Build history of the part. All positions in model axes, mm. A direction names the side the tool comes from. Give positions to 0.01 mm unless a question says otherwise; leave off trailing zeros. Write each loop counter-clockwise with the first axis right and the second up, starting at its lowest first coordinate (ties: lowest second). Pieces come first, ordered by that corner, then holes.
Autodesk Inventor part; units mm, degrees
ref_plane "YZ Plane" through (0, 0, 0) normal (1, 0, 0) x (0, 1, 0)
ref_plane "XZ Plane" through (0, 0, 0) normal (0, 1, 0) x (-1, 0, 0)
ref_plane "XY Plane" through (0, 0, 0) normal (0, 0, 1) x (1, 0, 0)
sketch "Sketch1" plane through (0, 0, 0) normal (1, 0, 0) x (0, 1, 0)
  line L0 (0, 0) -> (5, 0)
  line L1 (5, 0) -> (5, 20)
  line L2 (5, 20) -> (0, 20)
  line L3 (0, 20) -> (0, 0)
  line L4 (-25, 100) -> (-30, 100)
  line L5 (-30, 100) -> (-30, 120)
  line L6 (-30, 120) -> (-25, 120)
  line L7 (-25, 120) -> (-25, 100)
  line L8 (5, 20) -> (-25, 100)
  line L9 (0, 20) -> (-30, 100)
  dimension "d0" = 5
  dimension "d1" = 20
  dimension "d2" = 5
  dimension "d3" = 20
  dimension "d4" = 35
  dimension "d5" = 120
extrude "Extrusion1" add sketch "Sketch1" along normal blind 40
sketch "Sketch2" plane through (0, 0, 0) normal (0, -1, 0) x (1, 0, 0)
  circle A0 centre (30, 10) radius 2.5
  circle A1 centre (10, 10) radius 2.5
  circle A2 centre (30, 110) radius 2.5
  circle A3 centre (10, 110) radius 2.5
  line L0 (40, 120) -> (40, 100)
  line L1 (0, 120) -> (40, 120)
  line L2 (0, 120) -> (0, 100)
  line L3 (0, 20) -> (0, 0)
  line L4 (40, 20) -> (40, 0)
  line L5 (0, 0) -> (40, 0)
  dimension "d8" = 5
  dimension "d9" = 5
  dimension "d10" = 5
  dimension "d11" = 5
  dimension "d12" = 10
  dimension "d13" = 10
  dimension "d14" = 10
  dimension "d15" = 10
  dimension "d16" = 10
  dimension "d17" = 10
  dimension "d18" = 10
  dimension "d19" = 10
extrude "Extrusion2" cut sketch "Sketch2" against normal mid plane 90
properties part number "BracketControlPannel"
1. Saw through at B-B on z = 10. Give the cut face in (x, y).
2. Drop a flat-ended pin along its axis: pin 1 (22 mm diameter, centred on x = 28.5, z = 6, fed in from -Y). Give the stop position or say it passes through.
3. Drill centre lines: line 1 along Y through (x, z) = (4, 17); line 2 along Y through (x, z) = (34, 103.5). Where is each one in solid material? Low to high.
4. Mould opens along Z. For faces 4 (the face through (20, 2, 0)), 5 (the face through (29.46, 2.46, 7.56)), 6 (the face through (9.46, 2.46, 7.56)), 7 (the face through (0, -13, 60)) say: pulls with the +Z half, pulls with the -Z half, needs draft (parallel to the pull), parting line crosses it, or undercut.
5. Saw through at C-C on x = 24. Give the cut face in (y, z).
6. Saw through at A-A on x = 30. Give the cut face in (y, z), plus the area to 3 significant figures.
7. 3-axis set-ups, long thin cutter, end or side, ignore diameter. For faces 1 (the face through (40, -13, 60)), 2 (the face through (20, 0, 10)), 3 (the face through (20, -25, 110)): which of +Z, -Z, +X, -X, +Y, -Y reach the whole face in a straight line?
8. Saw through at D-D on z = 96.5. Give the cut face in (x, y).
Outcome:
1. outline: (0, 0) - (7.5, 0) - (7.5, 5) - (0, 5) - close; (12.5, 0) - (27.5, 0) - (27.5, 5) - (12.5, 5) - close; (32.5, 0) - (40, 0) - (40, 5) - (32.5, 5) - close
2. pin 1: stops at y = 0
3. line 1: y = 0 to 5
3. line 2: y = -30 to -25
4. face 4: pulls with the -Z half
4. face 5: undercut
4. face 6: undercut
4. face 7: needs draft
5. outline: (-30, 100) - (0, 20) - (0, 0) - (5, 0) - (5, 20) - (-25, 100) - (-25, 120) - (-30, 120) - close
6. outline: (-30, 100) - (0, 20) - (0, 12.5) - (5, 12.5) - (5, 20) - (-25, 100) - (-25, 107.5) - (-30, 107.5) - close; (-30, 112.5) - (-25, 112.5) - (-25, 120) - (-30, 120) - close; (0, 0) - (5, 0) - (5, 7.5) - (0, 7.5) - close
6. area: 550 mm2
7. face 1: +Z, -Z, +X, +Y, -Y
7. face 2: -Z, +X, -X, -Y
7. face 3: +Z, +X, -X, +Y
8. outline: (0, -28.69) - (40, -28.69) - (40, -23.69) - (0, -23.69) - close
